Source: CAD feature listing. Evaluate the final solid. Frame: model axes, mm. A direction names the side the tool comes from. Give positions to 0.01 mm unless a question says otherwise; leave off trailing zeros. Write each loop counter-clockwise with the first axis right and the second up, starting at its lowest first coordinate (ties: lowest second). Pieces come first, ordered by that corner, then holes. Notation, with made-up numbers: (51.25, -17.5) -> (65.25, -17.5) arc R30 cw to (65.25, 19.5) -> close; hole circle Ø5 at (20, 35.25). An arc over 180 degrees is marked (long way). Use one line per item in the form item = value. Start each with the question number.
(1) Set-up query: faces 1 (the face through (6.979, 37.966, 21.74)), 2 (the face through (-4, 26, 24.2)), 3 (the face through (0, 23.7, 27)), 4 (the face through (-6, 32, 22.5)), 5 (the face through (-18.05, 26, 28)). Return all of +Z, -Z, +X, -X, +Y, -Y with unobstructed straight access to the full face (end or side cutting, diameter ignored); none if empty.
(2) First-contact query: P1, Ø1.5, axis at x = -6, z = 23.5, coming from the +Y side; P2, Ø3.5, axis at y = 27, z = 22.5, coming from the -X side; P3, Ø1.5, axis at y = 34.5, z = 20, coming from the -X side; P4, Ø3, axis at x = 0, y = 20, coming from the -Z side. Flat tips, straight axial feed; report the tip coordinate or a pass-through.
(3) Cut plane D-D, the plane x = 4. Output: boundary loops of the cut face in (y, z).
(4) Cut plane B-B, the plane x = -12.5. Output: boundary loops of the cut face in (y, z), and give its area (3 significant figures).
(5) Draft query along Z for faces 6 (the face through (-15.05, 26, 23)), 7 (the face through (15.858, 26.165, 35.883)), 8 (the face through (-8.021, 37.966, 21.74)). Return one class per face: pulls with the +Z half, pulls with the -Z half, needs draft (parallel to the pull), parting line crosses it, or undercut.
(6) Cut plane A-A, the plane y = 34. Output: boundary loops of the cut face in (x, z).
(7) Material intervals for line 1 along X through (y, z) = (28, 23); line 2 along Y through (x, z) = (-7.5, 22); line 3 along Y through (x, z) = (0, 19), sorted ascending. Write a range as from..to.
(8) Cut plane C-C, the plane z = 32.75. Output: boundary loops of the cut face in (x, y), and give its area (3 significant figures).
from build123d import *

# Parameters (mm, degrees)
CYLINDER006_R                   = 1.6
CYLINDER006_DEPTH               = 10
BOX007_W                        = 3.1
BOX007_H                        = 5
BOX007_DEPTH                    = 8
BOX009_W                        = 3.1
BOX009_H                        = 5
BOX009_DEPTH                    = 9
BOX010_W                        = 3.1
BOX010_H                        = 5
BOX010_DEPTH                    = 9
BOX012_W                        = 31
BOX012_H                        = 6
BOX012_DEPTH                    = 6
CYLINDER004_R                   = 21.5
CYLINDER004_DEPTH               = 10
BOX008_W                        = 30.1
BOX008_H                        = 5
BOX008_DEPTH                    = 18
FILLET001003_R                  = 1
FILLET001007_R                  = 1
CYLINDER003_R                   = 18.5
CYLINDER003_DEPTH               = 10
BOX005_W                        = 36.1
BOX005_H                        = 5
BOX005_DEPTH                    = 18
FILLET001004_R                  = 1
CYLINDER010_R                   = 2
CYLINDER010_DEPTH               = 4.5
CYLINDER011_R                   = 2
CYLINDER011_DEPTH               = 4.5
CYLINDER008_R                   = 4
CYLINDER008_DEPTH               = 4.5
BOX011_W                        = 28.1
BOX011_H                        = 12
BOX011_DEPTH                    = 3
FILLET001006_R                  = 2
CYLINDER009_R                   = 4
CYLINDER009_DEPTH               = 4.5
BOX006_W                        = 44.1
BOX006_H                        = 15.6
BOX006_DEPTH                    = 3
FILLET001005_R                  = 1
CHAMFER005021077002006002_SIZE2 = 14
CHAMFER005021077002006002_SIZE  = 4
CHAMFER005021077002006003_SIZE2 = 14
CHAMFER005021077002006003_SIZE  = 4


with BuildPart() as cylinder006:
    # Cylinder006 → Cylinder006 (new body)
    with BuildSketch(Plane(origin=(0, 20, 18), x_dir=(1, 0, 0), z_dir=(0, 0, 1))):
        Circle(CYLINDER006_R)
    extrude(amount=CYLINDER006_DEPTH)


with BuildPart() as cube007:
    # Box007 → Box007 (new body)
    with BuildSketch(Plane(origin=(-1.55, 13.5, 18), x_dir=(1, 0, 0), z_dir=(0, 0, 1))):
        with Locations((1.55, 2.5)):
            Rectangle(BOX007_W, BOX007_H)
    extrude(amount=BOX007_DEPTH)


with BuildPart() as cube009:
    # Box009 → Box009 (new body)
    with BuildSketch(Plane(origin=(-9.55, 13.5, 18), x_dir=(1, 0, 0), z_dir=(0, 0, 1))):
        with Locations((1.55, 2.5)):
            Rectangle(BOX009_W, BOX009_H)
    extrude(amount=BOX009_DEPTH)


with BuildPart() as fusion036012039011002025018010027010:
    # Box010 → Box010 (new body)
    with BuildSketch(Plane(origin=(6.45, 13.5, 18), x_dir=(1, 0, 0), z_dir=(0, 0, 1))):
        with Locations((1.55, 2.5)):
            Rectangle(BOX010_W, BOX010_H)
    extrude(amount=BOX010_DEPTH)

    # Fusion036012039011002025018010027010: union Cube007, Cube009
    add(cube007.part)
    add(cube009.part)


with BuildPart() as fusion036012039011002025018010027011:
    # Box012 → Box012 (new body)
    with BuildSketch(Plane(origin=(-15.5, 13.2, 24.2), x_dir=(1, 0, 0), z_dir=(0, 0, 1))):
        with Locations((15.5, 3)):
            Rectangle(BOX012_W, BOX012_H)
    extrude(amount=BOX012_DEPTH)

    # Fusion036012039011002025018010027011: union Fusion036012039011002025018010027010
    add(fusion036012039011002025018010027010.part)


with BuildPart() as cylinder004:
    # Cylinder004 → Cylinder004 (new body)
    with BuildSketch(Plane(origin=(0, 10.3, 45.66), x_dir=(1, 0, 0), z_dir=(0, 1, 0))):
        Circle(CYLINDER004_R)
    extrude(amount=CYLINDER004_DEPTH)


with BuildPart() as fillet001007:
    # Box008 → Box008 (new body)
    with BuildSketch(Plane(origin=(-15.05, 13.5, 21), x_dir=(1, 0, 0), z_dir=(0, 0, 1))):
        with Locations((15.05, 2.5)):
            Rectangle(BOX008_W, BOX008_H)
    extrude(amount=BOX008_DEPTH)

    # Cut003: cut Cylinder004
    add(cylinder004.part, mode=Mode.SUBTRACT)

    # Fillet001003
    fillet001003_edges = [fillet001007.edges().sort_by_distance(p)[0] for p in [
        (-15.05, 16, 30.305929),
        (-15.05, 16, 21),
        (15.05, 16, 30.305929),
        (15.05, 16, 21),
    ]]
    fillet(fillet001003_edges, radius=FILLET001003_R)

    # Cut005003: cut Fusion036012039011002025018010027011
    add(fusion036012039011002025018010027011.part, mode=Mode.SUBTRACT)

    # Fillet001007
    fillet001007_edges = [fillet001007.edges().sort_by_distance(p)[0] for p in [
        (-15.05, 16, 24.2),
        (15.05, 16, 24.2),
    ]]
    fillet(fillet001007_edges, radius=FILLET001007_R)


with BuildPart() as cylinder003:
    # Cylinder003 → Cylinder003 (new body)
    with BuildSketch(Plane(origin=(0, 10.3, 45.66), x_dir=(1, 0, 0), z_dir=(0, 1, 0))):
        Circle(CYLINDER003_R)
    extrude(amount=CYLINDER003_DEPTH)


with BuildPart() as cut005004:
    # Box005 → Box005 (new body)
    with BuildSketch(Plane(origin=(-18.05, 13.5, 18), x_dir=(1, 0, 0), z_dir=(0, 0, 1))):
        with Locations((18.05, 2.5)):
            Rectangle(BOX005_W, BOX005_H)
    extrude(amount=BOX005_DEPTH)

    # Cut002: cut Cylinder003
    add(cylinder003.part, mode=Mode.SUBTRACT)

    # Fillet001004
    fillet001004_edges = [cut005004.edges().sort_by_distance(p)[0] for p in [
        (-18.05, 16, 36),
        (-15.777655, 16, 36),
        (18.05, 16, 36),
        (15.777655, 16, 36),
    ]]
    fillet(fillet001004_edges, radius=FILLET001004_R)

    # Cut005004: cut Fillet001007
    add(fillet001007.part, mode=Mode.SUBTRACT)


with BuildPart() as cut005004_1:
    # Cut005004 placement: moved
    add(cut005004.part.moved(Location((0, 10.2, 0))))


with BuildPart() as cylinder010:
    # Cylinder010 → Cylinder010 (new body)
    with BuildSketch(Plane(origin=(7.5, 34, 18), x_dir=(1, 0, 0), z_dir=(0, 0, 1))):
        Circle(CYLINDER010_R)
    extrude(amount=CYLINDER010_DEPTH)


with BuildPart() as fusion036012039011002025018010027009:
    # Cylinder011 → Cylinder011 (new body)
    with BuildSketch(Plane(origin=(-7.5, 34, 18), x_dir=(1, 0, 0), z_dir=(0, 0, 1))):
        Circle(CYLINDER011_R)
    extrude(amount=CYLINDER011_DEPTH)

    # Fusion036012039011002025018010027009: union Cylinder010
    add(cylinder010.part)


with BuildPart() as cylinder008:
    # Cylinder008 → Cylinder008 (new body)
    with BuildSketch(Plane(origin=(-7.5, 34, 18), x_dir=(1, 0, 0), z_dir=(0, 0, 1))):
        Circle(CYLINDER008_R)
    extrude(amount=CYLINDER008_DEPTH)


with BuildPart() as fillet001006:
    # Box011 → Box011 (new body)
    with BuildSketch(Plane(origin=(-14.05, 28, 18), x_dir=(1, 0, 0), z_dir=(0, 0, 1))):
        with Locations((14.05, 6)):
            Rectangle(BOX011_W, BOX011_H)
    extrude(amount=BOX011_DEPTH)

    # Fillet001006
    fillet001006_edges = [fillet001006.edges().sort_by_distance(p)[0] for p in [
        (-14.05, 40, 19.5),
        (14.05, 40, 19.5),
    ]]
    fillet(fillet001006_edges, radius=FILLET001006_R)


with BuildPart() as cut005002:
    # Cylinder009 → Cylinder009 (new body)
    with BuildSketch(Plane(origin=(7.5, 34, 18), x_dir=(1, 0, 0), z_dir=(0, 0, 1))):
        Circle(CYLINDER009_R)
    extrude(amount=CYLINDER009_DEPTH)

    # Fusion036012039011002025018010027008: union Cylinder008, Fillet001006
    add(cylinder008.part)
    add(fillet001006.part)

    # Cut005002: cut Fusion036012039011002025018010027009
    add(fusion036012039011002025018010027009.part, mode=Mode.SUBTRACT)


with BuildPart() as cut005005:
    # Box006 → Box006 (new body)
    with BuildSketch(Plane(origin=(-22.05, 13.1, 18), x_dir=(1, 0, 0), z_dir=(0, 0, 1))):
        with Locations((22.05, 7.8)):
            Rectangle(BOX006_W, BOX006_H)
    extrude(amount=BOX006_DEPTH)

    # Fillet001005
    fillet001005_edges = [cut005005.edges().sort_by_distance(p)[0] for p in [
        (-22.05, 13.1, 19.5),
        (22.05, 13.1, 19.5),
    ]]
    fillet(fillet001005_edges, radius=FILLET001005_R)

    # Chamfer005021077002006002
    chamfer005021077002006002_edges = [cut005005.edges().sort_by_distance(p)[0] for p in [
        (22.05, 28.7, 19.5),
    ]]
    chamfer005021077002006002_side = cut005005.faces().sort_by_distance((0, 28.7, 19.5))[0]
    chamfer(chamfer005021077002006002_edges, length=CHAMFER005021077002006002_SIZE, length2=CHAMFER005021077002006002_SIZE2, reference=chamfer005021077002006002_side)

    # Chamfer005021077002006003
    chamfer005021077002006003_edges = [cut005005.edges().sort_by_distance(p)[0] for p in [
        (-22.05, 28.7, 19.5),
    ]]
    chamfer005021077002006003_side = cut005005.faces().sort_by_distance((-2, 28.7, 19.5))[0]
    chamfer(chamfer005021077002006003_edges, length=CHAMFER005021077002006003_SIZE, length2=CHAMFER005021077002006003_SIZE2, reference=chamfer005021077002006003_side)

    # Fusion036012039011002025018010027012: union Cut005004, Cut005002
    add(cut005004_1.part)
    add(cut005002.part)

    # Cut005005: cut Cylinder006
    add(cylinder006.part, mode=Mode.SUBTRACT)


solid = cut005005.part
Geometry says:
q1.face_1 = +Z
q1.face_2 = +Y, -Y
q1.face_3 = +Z, +X, -X, -Y
q1.face_4 = +Z, +X, -X, +Y
q1.face_5 = +Z, -X, +Y, -Y
q2.P1 = 28.7
q2.P2 = -18.79
q2.P3 = -14.05
q2.P4 = through
q3.outline = (13.1, 18) -> (40, 18) -> (40, 21) -> (35.94, 21) -> (35.94, 22.5) -> (32.06, 22.5) -> (32.06, 21) -> (13.1, 21) -> close; (23.7, 24.2) -> (28.7, 24.2) -> (28.7, 27.6) -> (23.7, 27.6) -> close
q4.outline = (13.1, 18) -> (39.95, 18) -> (39.95, 21) -> (13.1, 21) -> close; (23.7, 24.2) -> (28.7, 24.2) -> (28.7, 32.02) -> (23.7, 32.02) -> close
q4.area = 120 mm^2
q5.face_6 = undercut
q5.face_7 = pulls with the +Z half
q5.face_8 = needs draft
q6.outline = (-14.05, 18) -> (-9.5, 18) -> (-9.5, 22.5) -> (-11.5, 22.5) -> (-11.5, 21) -> (-14.05, 21) -> close; (-5.5, 18) -> (5.5, 18) -> (5.5, 22.5) -> (3.5, 22.5) -> (3.5, 21) -> (-3.5, 21) -> (-3.5, 22.5) -> (-5.5, 22.5) -> close; (9.5, 18) -> (14.05, 18) -> (14.05, 21) -> (11.5, 21) -> (11.5, 22.5) -> (9.5, 22.5) -> close
q7.line_1 = -18.05..-15.05, -9.55..-6.45, -1.55..1.55, 6.45..9.55, 15.05..18.05
q7.line_2 = 23.7..28.7, 30..32, 36..38
q7.line_3 = 13.1..18.4, 21.6..40
q8.outline = (-18.05, 23.7) -> (-13.25, 23.7) -> (-13.25, 28.7) -> (-18.05, 28.7) -> close; (13.25, 23.7) -> (18.05, 23.7) -> (18.05, 28.7) -> (13.25, 28.7) -> close
q8.area = 48.0 mm^2
